from build123d import *

# Parameters (mm, degrees)
F1_DEPTH  = 600
F2_T      = -5
F4_DEPTH  = 25
F5_W      = 300
F5_H      = 75
F5_W_2    = 280
F5_H_2    = 55
F6_DEPTH  = 25
F7_W      = 870
F7_H      = 30
F8_DEPTH  = 15
F9_W      = 142.9338163137
F9_H      = 217.2664716095
F10_DEPTH = 18
F12_DEPTH = 12
F13_R     = 24.8551421214
F14_DEPTH = 5
F16_DEPTH = 10
F18_DEPTH = 870
F20_DEPTH = 20
F22_DEPTH = 18
F25_DEPTH = 5
F27_DEPTH = 5
F28_W     = 391.7387041664
F28_H     = 69.7681009769
F28_W_2   = 377.2408955904
F29_DEPTH = 25
F30_R     = 112.5
F31_DEPTH = 422
F32_W     = 900
F32_H     = 625
F32_R     = 112.5
F33_DEPTH = 20


with BuildPart() as f1:
    # F0 (on Front) → F1 (new body)
    with BuildSketch(Plane.XZ):
        with BuildLine():
            Line((-450, -750), (450, -750))
            Line((450, -750), (450, 750))
            ThreePointArc((450, 750), (0, 856.9714450254), (-450, 750))
            Line((-450, 750), (-450, -750))
        make_face()
    extrude(amount=F1_DEPTH)

    # F2
    f2_openings = [f1.faces().sort_by_distance(p)[0] for p in [
        (0, 0, 36.375009),
    ]]
    offset(amount=F2_T, openings=f2_openings)

    # F3 (on face) → F4 (join)
    with BuildSketch(Plane.XZ.offset(600)):
        with BuildLine():
            Line((450, -750), (450, 750))
            ThreePointArc((450, 750), (0, 856.9714450254), (-450, 750))
            Line((-450, 750), (-450, -750))
            Line((-450, -750), (450, -750))
        make_face()
        with BuildLine():
            Line((435, 740.7134888368), (435, -735))
            Line((435, -735), (-435, -735))
            Line((-435, -735), (-435, 740.7134888368))
            ThreePointArc((-435, 740.7134888368), (0, 841.9714450254), (435, 740.7134888368))
        make_face(mode=Mode.SUBTRACT)
    extrude(amount=F4_DEPTH)

    # F5 (on face) → F6 (join)
    with BuildSketch(Plane.XZ.offset(600)):
        with Locations((-200.8810852704, 318.7295198674)):
            Rectangle(F5_W, F5_H)
        with Locations((-200.8810852704, 318.7295198674)):
            Rectangle(F5_W_2, F5_H_2, mode=Mode.SUBTRACT)
        with Locations((211.2015885351, 318.7295198674)):
            Rectangle(F5_W, F5_H)
        with Locations((211.2015885351, 318.7295198674)):
            Rectangle(F5_W_2, F5_H_2, mode=Mode.SUBTRACT)
    extrude(amount=F6_DEPTH)

    # F7 (on face) → F8 (join)
    with BuildSketch(Plane.XZ.offset(600)):
        with Locations((0, 170.2089005709)):
            Rectangle(F7_W, F7_H)
    extrude(amount=F8_DEPTH)

    # F9 (on face) → F10 (join)
    with BuildSketch(Plane.XZ.offset(600)):
        Polygon((-14.5836101339, 155.2089005709), (-22.9078065604, 155.2089005709), (-22.9078065604, 42.8976975381), (-69.0468810499, 42.8976975381), (-69.0468810499, -194.3687740713), (93.8869352639, -194.3687740713), (93.8869352639, 42.8976975381), (44.0564386487, 42.8976975381), (44.0564386487, 155.2089005709), (34.6765947954, 155.2089005709), (34.6765947954, 42.8976975381), (-14.5836101339, 42.8976975381), align=None)
        with Locations((12.420027107, -75.7355382666)):
            Rectangle(F9_W, F9_H, mode=Mode.SUBTRACT)
    extrude(amount=F10_DEPTH)

    # F11 (on face) → F12 (join)
    with BuildSketch(Plane.XZ.offset(600)):
        Polygon((-22.9078065604, 155.2089005709), (-408.6377620697, 155.2089005709), (-408.6377620697, -707.8300118446), (408.7606370449, -707.8300118446), (408.7606370449, 155.2089005709), (44.0564386487, 155.2089005709), (44.0564386487, 42.8976975381), (93.8869352639, 42.8976975381), (93.8869352639, -194.3687740713), (-69.0468810499, -194.3687740713), (-69.0468810499, 42.8976975381), (-22.9078065604, 42.8976975381), align=None)
    extrude(amount=F12_DEPTH)

    # F13 (on face) → F14 (join)
    with BuildSketch(Plane.XZ.offset(612)):
        with Locations((-354.0675938129, -333.6301445961)):
            Circle(F13_R)
    extrude(amount=F14_DEPTH)

    # F15 (on face) → F16 (join)
    with BuildSketch(Plane.XZ.offset(612)):
        Polygon((-387.899610247, -268.6794745922), (-316.3461361468, -268.6794745922), (-353.5931451269, -212.8089411077), align=None)
        Polygon((-378.9620697498, -263.6794745922), (-353.4200489521, -222.0824658871), (-325.6887197495, -263.6794745922), align=None, mode=Mode.SUBTRACT)
    extrude(amount=F16_DEPTH)

    # F17 (on face) → F18 (join, through all)
    with BuildSketch(Plane.YZ.offset(-435)):
        with BuildLine():
            Line((-625, 577.9839080805), (-625, 586.1312416531))
            ThreePointArc((-625, 586.1312416531), (-667.0829642918, 573.1979535583), (-705.2572369576, 551.2669086456))
            Line((-705.2572369576, 551.2669086456), (-693.4141296704, 549.7889105873))
            ThreePointArc((-693.4141296704, 549.7889105873), (-660.5960632562, 567.2567631744), (-625, 577.9839080805))
        make_face()
        with BuildLine():
            Line((-600, 581.2005341429), (-600, 589.2150402069))
            ThreePointArc((-600, 589.2150402069), (-612.5491949312, 588.0719585758), (-625, 586.1312416531))
            Line((-625, 586.1312416531), (-625, 577.9839080805))
            ThreePointArc((-625, 577.9839080805), (-612.5535193278, 580.008179687), (-600, 581.2005341429))
        make_face()
    extrude(amount=F18_DEPTH)

    # F19 (on face) → F20 (join)
    with BuildSketch(Plane.YZ.offset(435)):
        with BuildLine():
            ThreePointArc((-625, 577.9839080805), (-660.5960632562, 567.2567631744), (-693.4141296704, 549.7889105873))
            Line((-693.4141296704, 549.7889105873), (-600, 538.1309986115))
            Line((-600, 538.1309986115), (-600, 589.2150402069))
            ThreePointArc((-600, 589.2150402069), (-612.5491949312, 588.0719585758), (-625, 586.1312416531))
            Line((-625, 586.1312416531), (-625, 577.9839080805))
        make_face()
        with BuildLine():
            ThreePointArc((-625, 586.1312416531), (-667.0829642918, 573.1979535583), (-705.2572369576, 551.2669086456))
            Line((-705.2572369576, 551.2669086456), (-693.4141296704, 549.7889105873))
            ThreePointArc((-693.4141296704, 549.7889105873), (-660.5960632562, 567.2567631744), (-625, 577.9839080805))
            Line((-625, 577.9839080805), (-625, 586.1312416531))
        make_face()
    extrude(amount=-F20_DEPTH)

    # F21 (on face) → F22 (join)
    with BuildSketch(Plane(origin=(-435, 0, 0), x_dir=(0, -1, 0), z_dir=(-1, 0, 0))):
        with BuildLine():
            ThreePointArc((625, 577.9839080805), (660.5960632562, 567.2567631744), (693.4141296704, 549.7889105873))
            Line((693.4141296704, 549.7889105873), (705.2572369576, 551.2669086456))
            ThreePointArc((705.2572369576, 551.2669086456), (667.0829642918, 573.1979535583), (625, 586.1312416531))
            Line((625, 586.1312416531), (625, 577.9839080805))
        make_face()
        with BuildLine():
            Line((600, 589.2150402069), (600, 581.2005341429))
            Line((600, 581.2005341429), (600, 538.1309986115))
            Line((600, 538.1309986115), (693.4141296704, 549.7889105873))
            ThreePointArc((693.4141296704, 549.7889105873), (660.5960632562, 567.2567631744), (625, 577.9839080805))
            Line((625, 577.9839080805), (625, 586.1312416531))
            ThreePointArc((625, 586.1312416531), (612.5491949312, 588.0719585758), (600, 589.2150402069))
        make_face()
    extrude(amount=-F22_DEPTH)

    # F24 (on offset) → F25 (join)
    with BuildSketch(Plane.YZ):
        with BuildLine():
            Line((-600, 538.1309986115), (-600, 581.2005341429))
            ThreePointArc((-600, 581.2005341429), (-648.7839740291, 571.6711832668), (-693.4141296704, 549.7889105873))
            Line((-693.4141296704, 549.7889105873), (-600, 538.1309986115))
        make_face()
    extrude(amount=F25_DEPTH)

    # F26 (on face) → F27 (join)
    with BuildSketch(Plane(origin=(0, 0, 0), x_dir=(-1, 0, 0), z_dir=(0, 1, 0))):
        with BuildLine():
            ThreePointArc((445, 746.9152634769), (0, 851.9714450254), (-445, 746.9152634769))
            Line((-445, 746.9152634769), (-445, -745))
            Line((-445, -745), (445, -745))
            Line((445, -745), (445, 746.9152634769))
        make_face()
    extrude(amount=-F27_DEPTH)

    # F28 (on face) → F29 (cut)
    with BuildSketch(Plane.XZ.offset(600)):
        with Locations((-207.7159030628, 527.7101248503)):
            Rectangle(F28_W, F28_H)
        with Locations((208.6599989108, 527.7101248503)):
            Rectangle(F28_W_2, F28_H)
    extrude(amount=-F29_DEPTH, mode=Mode.SUBTRACT)

    # F30 (on face) → F31 (join)
    with BuildSketch(Plane(origin=(0, 0, -750), x_dir=(1, 0, 0), z_dir=(0, 0, -1))):
        with Locations((0, 312.5)):
            Circle(F30_R)
    extrude(amount=F31_DEPTH)

    # F32 (on face) → F33 (join)
    with BuildSketch(Plane(origin=(0, 0, -1172), x_dir=(1, 0, 0), z_dir=(0, 0, -1))):
        with Locations((0, 312.5)):
            Rectangle(F32_W, F32_H)
        with Locations((0, 312.5)):
            Circle(F32_R, mode=Mode.SUBTRACT)
        with Locations((0, 312.5)):
            Circle(F32_R)
    extrude(amount=F33_DEPTH)


solid = f1.part
Part model, mm, in its own coordinate system. A direction names the side the tool comes from. Coordinates: 2 decimals unless noted, no trailing zeros. Loops run counter-clockwise (first coordinate to the right, second up) from the corner with the lowest first, then second, coordinate; pieces in that order, holes last. Notation, with made-up numbers: M -37,79.5 L -29,79.5 A14 ccw -29,96.5 Z; hole C -8.75,77 d7. An arc over 180 degrees is marked long. Use a Markdown table: item, result. Add a question column.
Q1. Cut at B-B (y = -312.5). Write the cut outline in (x, z), and give its area (3 significant figures).
Q2. Mould opens along Z. For faces 1 (the flat face through (450, -308, -10)), 2 (the flat face through (-6, -317, -1192)), 3 (the flat face through (-2, -600, -716)) say: +Z half, -Z half, draft (parallel to the pull), parting line (faces both ways), or undercut.
Q3. Cut at C-C (z = -890.5). Write the cut outline in (x, y).
Q4. Cut at A-A (y = -101.5). Write the cut outline in (x, z).
Q5. Probe L1, parallel to X at y = -205.5, z = 134; L2, parallel to Z at x = 22, y = -543.5; L3, parallel to Z at x = 363.5, y = -81. List the from-to ranges inside material, lowest first.
Q6. Pin check, flat tips, straight feed: P1, Ø3, axis at x = 111.5, z = 347.5, coming from the -Y side; P2, Ø4.5, axis at x = 112, y = -607.5, coming from the +Z side; P3, Ø2.5, axis at x = -174, y = -597, coming from the +Z side. Stop position of each tip, or through.
Q7. Which spindle directions (+Z, -Z, +X, -X, +Y, -Y) get a long thin tool onto all of the face, cutting with end or side? Do faces 4 (the cylindrical face through (6.46, -295.87, 851.95)), 5 (the flat face through (6, 0, 65)), 6 (the flat face through (-450, -308, 10)), 7 (the cylindrical face through (-6.31, -612.33, 841.95)), 8 (the flat face through (-202, -625, 347)). Say none if no direction does.
Worked out:
| question | item | result |
|---|---|---|
| 1 | outline | M -450,-1192 L 450,-1192 L 450,-1172 L 112.5,-1172 L 112.5,-750 L 450,-750 L 450,750 A1000 ccw -450,750 L -450,-750 L -112.5,-750 L -112.5,-1172 L -450,-1172 Z; hole M -445,-745 L 445,-745 L 445,746.92 A995 ccw -445,746.92 Z |
| 1 | area | 137,000 mm2 |
| 2 | face 1 | draft |
| 2 | face 2 | -Z half |
| 2 | face 3 | undercut |
| 3 | outline | C 0,-312.5 d225 |
| 4 | outline | M -450,-1192 L 450,-1192 L 450,-1172 L -450,-1172 Z; M -450,-750 L 450,-750 L 450,750 A1000 ccw -450,750 Z; hole M -445,-745 L 445,-745 L 445,746.92 A995 ccw -445,746.92 Z |
| 5 | L1 | x = -450 to -445, 445 to 450 |
| 5 | L2 | z = -1192 to -1172, -750 to -745, 851.73 to 856.73 |
| 5 | L3 | z = -1192 to -1172, -750 to -745, 783.2 to 788.57 |
| 6 | P1 | stops at y = -625 |
| 6 | P2 | stops at z = 850.93 |
| 6 | P3 | stops at z = 841.94 |
| 7 | face 4 | none |
| 7 | face 5 | +Z, -Z, +X, -X, +Y |
| 7 | face 6 | +Z, -Z, -X, +Y, -Y |
| 7 | face 7 | -Y |
| 7 | face 8 | -Z, +X, -X, -Y |
